```python
from build123d import *

# Parameters (mm, degrees)
SKETCH1_R           = 18.25
BOSS_EXTRUDE1_DEPTH = 26
CUT_EXTRUDE1_START  = -22
SKETCH2_R           = 18.25
SKETCH2_R_2         = 14
CUT_EXTRUDE1_DEPTH  = 22
SKETCH3_R           = 5
CUT_EXTRUDE2_DEPTH  = 37.635024225


with BuildPart() as part:
    # Sketch1 → Boss-Extrude1 (new body)
    with BuildSketch(Plane(origin=(0, 0, 0), x_dir=(1, 0, 0), z_dir=(0, 1, 0))):
        with Locations(Location((0, 0, 0), (0, 0, 90))):
            Circle(SKETCH1_R)
    extrude(amount=BOSS_EXTRUDE1_DEPTH)

    # Sketch2 → Cut-Extrude1 (cut)
    with BuildSketch(Plane(origin=(0, 26, 0), x_dir=(1, 0, 0), z_dir=(0, 1, 0)).offset(CUT_EXTRUDE1_START)):
        with Locations(Location((0, 0, 0), (0, 0, 90))):
            Circle(SKETCH2_R)
        with Locations(Location((0, 0, 0), (0, 0, 270))):
            Circle(SKETCH2_R_2, mode=Mode.SUBTRACT)
    extrude(amount=CUT_EXTRUDE1_DEPTH, mode=Mode.SUBTRACT)

    # Sketch3 → Cut-Extrude2 (cut, through all)
    with BuildSketch(Plane(origin=(0, 26, 0), x_dir=(1, 0, 0), z_dir=(0, 1, 0))):
        with Locations(Location((0, 0, 0), (0, 0, 270))):
            Circle(SKETCH3_R)
    extrude(amount=-CUT_EXTRUDE2_DEPTH, mode=Mode.SUBTRACT)

    # Sketch4 → Cut-Revolve1 (revolve, cut)
    with BuildSketch(Plane(origin=(0, 0, 0), x_dir=(0, 0, -1), z_dir=(1, 0, 0))):
        Polygon((-14, 24.4), (-14, 26), (-12.4, 26), align=None)
    revolve(axis=Axis((0, -1000, 0), (0, 1, 0)), mode=Mode.SUBTRACT)


solid = part.part
```
Could you check a few things on this model? Use its own coordinates, in mm. A direction names the side the tool comes from. Give positions to 0.01 mm unless a question says otherwise; leave off trailing zeros. Write each loop counter-clockwise with the first axis right and the second up, starting at its lowest first coordinate (ties: lowest second). Pieces come first, ordered by that corner, then holes. Notation, with made-up numbers: (86, 41.25) - (129, 41.25) arc R19 ccw to (129, 73.25) - close; hole circle Ø10 at (54.25, -17). An arc over 180 degrees is marked (long way). One line per item, written item: value. Start each with the question number.
Item 1: Imagine slicing it at A-A, the plane z = 0. List the corners of the cut face in (x, y) for me, and give its area (3 significant figures).
Item 2: Imagine slicing it at B-B, the plane x = 0. List the corners of the cut face in (y, z) for me.
Item 3: Imagine slicing it at C-C, the plane y = 2.75. List the corners of the cut face in (x, z) for me.
Item 4: If we mould it in two halves opening along X, with no side actions, what happens to faces 1 (the face through (-4.88, 13.18, -1.08)), 2 (the face through (-0.2, 26, -5.3)), 3 (the face through (-13.67, 14.06, -3.03))? For each: +X half, -X half, draft (parallel to the pull), parting line (faces both ways), or undercut.
Item 5: Which directions (+Z, -Z, +X, -X, +Y, -Y) give clear straight access to the entire face, cutting with the end or side of a thin tool? Please do faces 4 (the face through (17.816, 1.972, 3.956)), 5 (the face through (11, 4, -9)).
Item 6: I'm going to push flat-ended pins straight in: pin 1 (12 mm diameter, centred on x = -8, y = 22, fed in from -Z); pin 2 (5 mm diameter, centred on y = 19.5, z = 13.5, fed in from +X); pin 3 (2 mm diameter, centred on y = 13.5, z = -2, fed in from +X). Where does each tip first touch, or does it pass through?
Item 7: Please list where these lines run through material, in increasing order: line 1 (X direction, y = 15.75, z = 0); line 2 (Y direction, x = 17, z = 6); line 3 (X direction, y = 23, z = -1.5). Write a range as from..to.
Item 8: Imagine slicing it at D-D, the plane y = 15.5. List the corners of the cut face in (x, z) for me, and give its area (3 significant figures).
Geometry says:
1. outline: (-18.25, 0) - (-5, 0) - (-5, 26) - (-12.4, 26) - (-14, 24.4) - (-14, 4) - (-18.25, 4) - close; (5, 0) - (18.25, 0) - (18.25, 4) - (14, 4) - (14, 24.4) - (12.4, 26) - (5, 26) - close
1. area: 499 mm^2
2. outline: (0, -18.25) - (4, -18.25) - (4, -14) - (24.4, -14) - (26, -12.4) - (26, -5) - (0, -5) - close; (0, 5) - (26, 5) - (26, 12.4) - (24.4, 14) - (4, 14) - (4, 18.25) - (0, 18.25) - close
3. outline: circle Ø36.5 at (0, 0); hole circle Ø10 at (0, 0)
4. face 1: undercut
4. face 2: draft
4. face 3: parting line
5. face 4: +Y, -Y
5. face 5: +Y
6. pin 1: z = -13.86
6. pin 2: x = 8.66
6. pin 3: x = 13.96
7. line 1: -14..-5, 5..14
7. line 2: 0..4
7. line 3: -13.92..-4.77, 4.77..13.92
8. outline: circle Ø28 at (0, 0); hole circle Ø10 at (0, 0)
8. area: 537 mm^2
